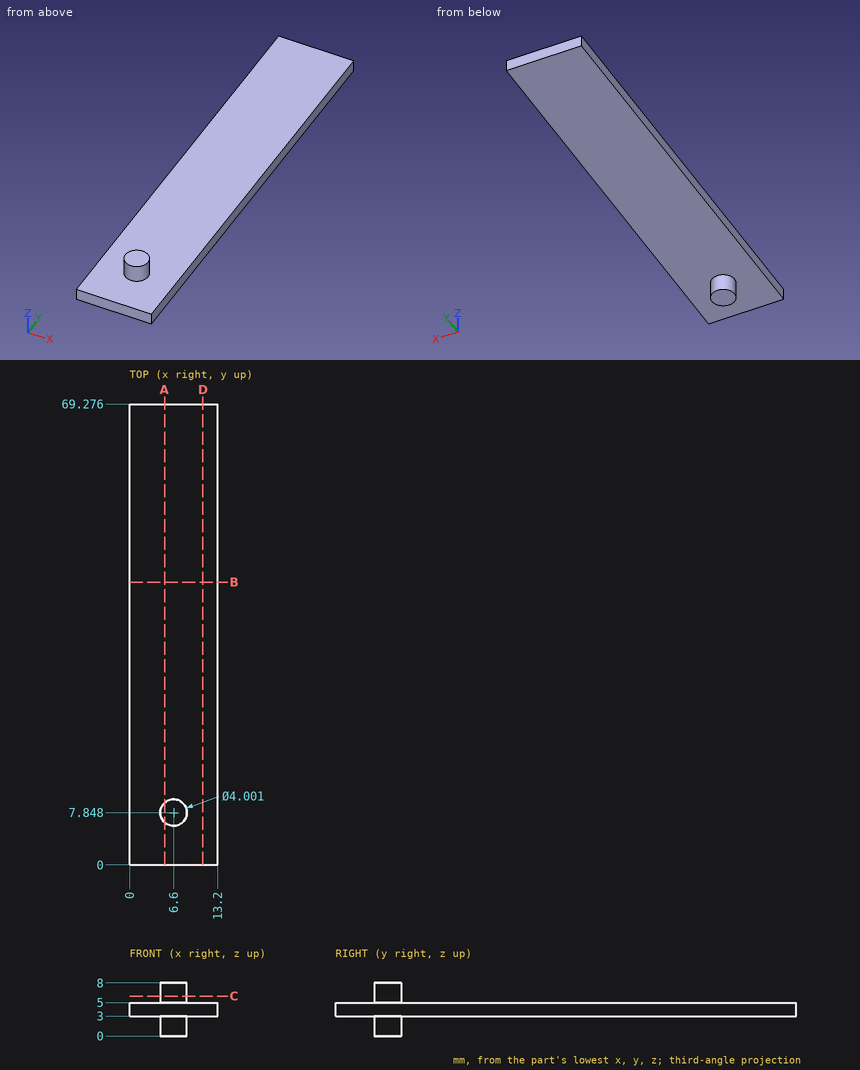
Check sheet for the drawn part. Datum: minimum x, y, z corner. Units: mm. Round coordinates to 2 decimals unless told otherwise and drop trailing zeros. Order: outer loops, then holes, each group sorted by start corner. A loop starts at its lowest first (then second) coordinate and runs counter-clockwise, first axis right, second up. Notation, with made-up numbers: (46, -30) - (81, -30) arc R19 ccw to (81, -9) - close; hole circle Ø4 at (68.5, -1). An arc over 180 degrees is marked (long way). Use a Markdown table: item, result. Add a question column.
(1) Sectioned sample at C-C, the plane z = 6. Enter the section's corners in (x, y).
(2) Sectioned sample at A-A, the plane x = 5.25. Enter the section's corners in (y, z) (1 decimal), and give its area (3 significant figures).
(3) Sectioned sample at D-D, the plane x = 11. Enter the section's corners in (y, z).
(4) Sectioned sample at B-B, the plane y = 42.5. Enter the section's corners in (x, z), and give its area (3 significant figures).
(5) Material ranges on line 1 along Z through (x, y) = (11, 25.5); line 2 along Y through (x, z) = (7, 7.75); line 3 along Y through (x, z) = (6.5, 2), recorded low to high. Write a range as [from, to].
Answers below:
| question | item | result |
|---|---|---|
| 1 | outline | circle Ø4 at (6.6, 7.85) |
| 2 | outline | (0, 3) - (6.4, 3) - (6.4, 0) - (9.3, 0) - (9.3, 3) - (69.3, 3) - (69.3, 5) - (9.3, 5) - (9.3, 8) - (6.4, 8) - (6.4, 5) - (0, 5) - close |
| 2 | area | 156 mm² |
| 3 | outline | (0, 3) - (69.28, 3) - (69.28, 5) - (0, 5) - close |
| 4 | outline | (0, 3) - (13.2, 3) - (13.2, 5) - (0, 5) - close |
| 4 | area | 26.4 mm² |
| 5 | line 1 | [3, 5] |
| 5 | line 2 | [5.89, 9.81] |
| 5 | line 3 | [5.85, 9.85] |
